The model under review builds one solid part; all positions refer to its coordinate system, in mm. A direction names the side the tool comes from. Coordinates: 2 decimals unless noted, no trailing zeros. Write each loop counter-clockwise with the first axis right and the second up, starting at its lowest first coordinate (ties: lowest second). Pieces come first, ordered by that corner, then holes. Notation, with made-up numbers: (35.25, 20.5) -> (43.25, 20.5) arc R17 cw to (43.25, 32.5) -> close; hole circle Ø1 at (5.25, -11). An arc over 180 degrees is marked (long way). Write each question's results on one line, items separated by ' | '.
```python
from build123d import *

# Parameters (mm, degrees)
SKIZZE1_W                                    = 110
SKIZZE1_H                                    = 60
AUFSATZ_LINEAR_AUSTRAGEN1_DEPTH              = 3
F_2_4_2_4_DURCHMESSER_BOHRUNG1_D             = 2.4
F_2_4_2_4_DURCHMESSER_BOHRUNG1_DEPTH         = 10
F_2_4_2_4_DURCHMESSER_BOHRUNG1_CSINK_D       = 2.45
F_2_4_2_4_DURCHMESSER_BOHRUNG1_CSINK_ANGLE   = 90
F_2_4_2_4_DURCHMESSER_BOHRUNG1_TIP           = 0.721032743
STIRNSENKUNG_F_R_M2_FLACHKOPFSCHRAUB_2_COUNT = 2
STIRNSENKUNG_F_R_M2_FLACHKOPFSCHRAUB_2_PITCH = 38.183766184
STIRNSENKUNG_F_R_M2_FLACHKOPFSCHRAUB_3_COUNT = 2
STIRNSENKUNG_F_R_M2_FLACHKOPFSCHRAUB_3_PITCH = 54
STIRNSENKUNG_F_R_M2_FLACHKOPFSCHRAUB_4_COUNT = 2
STIRNSENKUNG_F_R_M2_FLACHKOPFSCHRAUB_4_PITCH = 73.593477972
STIRNSENKUNG_F_R_M2_FLACHKOPFSCHRAUB_5_COUNT = 2
STIRNSENKUNG_F_R_M2_FLACHKOPFSCHRAUB_5_PITCH = 81.596568555
STIRNSENKUNG_F_R_M2_FLACHKOPFSCHRAUB_6_COUNT = 2
STIRNSENKUNG_F_R_M2_FLACHKOPFSCHRAUB_6_PITCH = 50
SKIZZE8_R                                    = 1
SKIZZE8_R_2                                  = 17.5
SCHNITT_LINEAR_AUSTRAGEN1_DEPTH              = 3


with BuildPart() as part:
    # Skizze1 → Aufsatz-Linear austragen1 (new body)
    with BuildSketch(Plane(origin=(0, 0, 0), x_dir=(1, 0, 0), z_dir=(0, 1, 0))):
        with Locations((55, 30)):
            Rectangle(SKIZZE1_W, SKIZZE1_H)
    extrude(amount=AUFSATZ_LINEAR_AUSTRAGEN1_DEPTH)

    # Ø2.4 (2.4) Durchmesser Bohrung1
    with Locations(Plane(origin=(0, 3, 0), x_dir=(1, 0, 0), z_dir=(0, 1, 0))):
        with Locations((30, 57), (80, 57), (107, 30), (80, 3), (30, 3), (3, 30), (133.088689194, 32.803420387)):
            CounterSinkHole(F_2_4_2_4_DURCHMESSER_BOHRUNG1_D / 2, F_2_4_2_4_DURCHMESSER_BOHRUNG1_CSINK_D / 2, depth=F_2_4_2_4_DURCHMESSER_BOHRUNG1_DEPTH, counter_sink_angle=F_2_4_2_4_DURCHMESSER_BOHRUNG1_CSINK_ANGLE)
            with Locations((0, 0, -(F_2_4_2_4_DURCHMESSER_BOHRUNG1_DEPTH + F_2_4_2_4_DURCHMESSER_BOHRUNG1_TIP / 2))):  # 118° drill point
                Cone(0, F_2_4_2_4_DURCHMESSER_BOHRUNG1_D / 2, F_2_4_2_4_DURCHMESSER_BOHRUNG1_TIP, mode=Mode.SUBTRACT)

    # Skizze7 → Stirnsenkung für M2 Flachkopfschraube mit Schlitz1 (revolve, cut)
    with BuildSketch(Plane(origin=(80, 3, -3), x_dir=(0, 0, 1), z_dir=(1, 0, 0))):
        Polygon((0, 0), (0, 2.721032743), (1.2, 2), (1.2, 1.6), (2.5, 1.6), (2.5, 0.025), (2.525, 0), align=None)
    stirnsenkung_f_r_m2_flachkopfschraube_mi = revolve(axis=Axis((80, 9.35, -3), (0, -1, 0)), mode=Mode.SUBTRACT)

    # Stirnsenkung f_r M2 Flachkopfschraub 2: Stirnsenkung für M2 Flachkopfschraube mit Schlitz1 ×2
    with Locations(*[Vector(0.7071067811865476, 0, -0.7071067811865476) * (i * STIRNSENKUNG_F_R_M2_FLACHKOPFSCHRAUB_2_PITCH) for i in range(1, STIRNSENKUNG_F_R_M2_FLACHKOPFSCHRAUB_2_COUNT)]):
        add(stirnsenkung_f_r_m2_flachkopfschraube_mi, mode=Mode.SUBTRACT)

    # Stirnsenkung f_r M2 Flachkopfschraub 3: Stirnsenkung für M2 Flachkopfschraube mit Schlitz1 ×2
    with Locations(*[(0, 0, -i * STIRNSENKUNG_F_R_M2_FLACHKOPFSCHRAUB_3_PITCH) for i in range(1, STIRNSENKUNG_F_R_M2_FLACHKOPFSCHRAUB_3_COUNT)]):
        add(stirnsenkung_f_r_m2_flachkopfschraube_mi, mode=Mode.SUBTRACT)

    # Stirnsenkung f_r M2 Flachkopfschraub 4: Stirnsenkung für M2 Flachkopfschraube mit Schlitz1 ×2
    with Locations(*[Vector(-0.6794080314983051, 0, -0.7337606740181692) * (i * STIRNSENKUNG_F_R_M2_FLACHKOPFSCHRAUB_4_PITCH) for i in range(1, STIRNSENKUNG_F_R_M2_FLACHKOPFSCHRAUB_4_COUNT)]):
        add(stirnsenkung_f_r_m2_flachkopfschraube_mi, mode=Mode.SUBTRACT)

    # Stirnsenkung f_r M2 Flachkopfschraub 5: Stirnsenkung für M2 Flachkopfschraube mit Schlitz1 ×2
    with Locations(*[Vector(-0.9436671340880456, 0, -0.33089626779710685) * (i * STIRNSENKUNG_F_R_M2_FLACHKOPFSCHRAUB_5_PITCH) for i in range(1, STIRNSENKUNG_F_R_M2_FLACHKOPFSCHRAUB_5_COUNT)]):
        add(stirnsenkung_f_r_m2_flachkopfschraube_mi, mode=Mode.SUBTRACT)

    # Stirnsenkung f_r M2 Flachkopfschraub 6: Stirnsenkung für M2 Flachkopfschraube mit Schlitz1 ×2
    with Locations(*[(-i * STIRNSENKUNG_F_R_M2_FLACHKOPFSCHRAUB_6_PITCH, 0, 0) for i in range(1, STIRNSENKUNG_F_R_M2_FLACHKOPFSCHRAUB_6_COUNT)]):
        add(stirnsenkung_f_r_m2_flachkopfschraube_mi, mode=Mode.SUBTRACT)

    # Skizze8 → Schnitt-Linear austragen1 (cut)
    with BuildSketch(Plane(origin=(0, 3, 0), x_dir=(1, 0, 0), z_dir=(0, 1, 0))):
        with Locations(Location((37.606134621, 42.637382924, 0), (0, 0, 270))):
            Circle(SKIZZE8_R)
        with Locations(Location((48.356134621, 50.4477151, 0), (0, 0, 270))):
            Circle(SKIZZE8_R)
        with Locations(Location((61.643865379, 50.4477151, 0), (0, 0, 270))):
            Circle(SKIZZE8_R)
        with Locations(Location((72.393865379, 42.637382924, 0), (0, 0, 270))):
            Circle(SKIZZE8_R)
        with Locations(Location((76.5, 30, 0), (0, 0, 270))):
            Circle(SKIZZE8_R)
        with Locations(Location((72.393865379, 17.362617076, 0), (0, 0, 270))):
            Circle(SKIZZE8_R)
        with Locations(Location((61.643865379, 9.5522849, 0), (0, 0, 270))):
            Circle(SKIZZE8_R)
        with Locations(Location((48.356134621, 9.5522849, 0), (0, 0, 270))):
            Circle(SKIZZE8_R)
        with Locations(Location((37.606134621, 17.362617076, 0), (0, 0, 270))):
            Circle(SKIZZE8_R)
        with Locations(Location((33.5, 30, 0), (0, 0, 270))):
            Circle(SKIZZE8_R)
        with Locations(Location((55, 30, 0), (0, 0, 270))):
            Circle(SKIZZE8_R_2)
    extrude(amount=-SCHNITT_LINEAR_AUSTRAGEN1_DEPTH, mode=Mode.SUBTRACT)


solid = part.part
```
Q1. For line 1 (Z direction, x = 80, y = 2.4); line 2 (Z direction, x = 30, y = 1.05); line 3 (X direction, y = 1.1, z = -18), list the stretches that pass through material, from the lowest coordinate up. Write a range as from..to.
Solution:
line 1: -60..-59.5, -54.5..-5.5, -0.5..0 | line 2: -60..-58.2, -55.8..-4.2, -1.8..0 | line 3: 0..36.84, 38.38..42.26, 67.74..71.62, 73.16..110
Q2. Add section A-A (z = -57). Write out the cut boundary in (x, y) (3 decimals).
Solution:
outline: (0, 0) -> (28.8, 0) -> (28.8, 1.4) -> (27.5, 1.4) -> (27.5, 2.975) -> (27.475, 3) -> (0, 3) -> close; (31.2, 0) -> (78.8, 0) -> (78.8, 1.4) -> (77.5, 1.4) -> (77.5, 2.975) -> (77.475, 3) -> (32.525, 3) -> (32.5, 2.975) -> (32.5, 1.4) -> (31.2, 1.4) -> close; (81.2, 0) -> (110, 0) -> (110, 3) -> (82.525, 3) -> (82.5, 2.975) -> (82.5, 1.4) -> (81.2, 1.4) -> close
Q3. Draft analysis for pull direction Z (two halves, no side actions). For faces 3 (the flat face through (110, 1, -30)), 4 (the flat face through (54, 1, 0)), 5 (the flat face through (29, 1.4, -4)), state which applies: pulls with the +Z half, pulls with the -Z half, needs draft (parallel to the pull), parting line crosses it, or undercut.
Solution:
face 3: needs draft | face 4: pulls with the +Z half | face 5: undercut
Q4. Clearance check with a flat-ended pin moving along its axis: P1, Ø2.5, axis at x = 80, z = -2.5, coming from the +Y side. State where the tip first meets the part, or that it passes through.
Solution:
P1: y = 1.4
Q5. Add section D-D (y = 2.2). Count the separate pieces of the cut face and the enclosed holes in it, plus the area to 3 significant figures.
Solution:
separate pieces: 1 | enclosed holes: 17 | area: 5,490 mm²
Q6. Add section C-C (x = 58.5). Write out the cut boundary in (y, z).
Solution:
outline: (0, -60) -> (3, -60) -> (3, -47.15) -> (0, -47.15) -> close; (0, -12.85) -> (3, -12.85) -> (3, 0) -> (0, 0) -> close
Q7. Machinability: for faces 1 (the cylindrical face through (105.855, 0.69, -30.36)), 2 (the flat face through (79, 1.4, -4)), which of the approach directions +Z, -Z, +X, -X, +Y, -Y give a long, thin tool a straight path to every point of the face, cutting with its end or side? Answer none if there is none.
Solution:
face 1: +Y, -Y | face 2: +Y
Q8. Add section B-B (x = 30). Write out the cut boundary in (y, z) (3 decimals).
Solution:
outline: (0, -60) -> (3, -60) -> (3, -59.525) -> (2.975, -59.5) -> (1.4, -59.5) -> (1.4, -58.2) -> (0, -58.2) -> close; (0, -55.8) -> (1.4, -55.8) -> (1.4, -54.5) -> (2.975, -54.5) -> (3, -54.475) -> (3, -5.525) -> (2.975, -5.5) -> (1.4, -5.5) -> (1.4, -4.2) -> (0, -4.2) -> close; (0, -1.8) -> (1.4, -1.8) -> (1.4, -0.5) -> (2.975, -0.5) -> (3, -0.475) -> (3, 0) -> (0, 0) -> close
